Model file for the job. Use its own axes, mm. Coordinates: 2 decimals unless noted, no trailing zeros. Write each loop counter-clockwise with the first axis right and the second up, starting at its lowest first coordinate (ties: lowest second). Pieces come first, ordered by that corner, then holes. Notation, with made-up numbers: M 20,24.25 L 62,24.25 A35 cw 62,60.25 Z; hole C -2.75,87.25 d1. An arc over 180 degrees is marked long. Use CSV: the item, a comma, the result in double quotes. Start each with the question number.
from build123d import *

# Parameters (mm, degrees)
BOSS_EXTRUDE1_DEPTH                       = 3.175
CSK_FOR_0_FLAT_HEAD_MACHINE_SCREW_2_COUNT = 2
CSK_FOR_0_FLAT_HEAD_MACHINE_SCREW_2_PITCH = 47.625
LPATTERN1_COUNT                           = 4
LPATTERN1_PITCH                           = 25.4
LPATTERN2_COUNT                           = 3
LPATTERN2_PITCH                           = 50.8


with BuildPart() as part:
    # Sketch1 → Boss-Extrude1 (new body)
    with BuildSketch(Plane.XY):
        with BuildLine():
            Line((0, 0), (0, 152.4))
            Line((0, 152.4), (-6.35, 152.4))
            ThreePointArc((-6.35, 152.4), (-10.840128061, 154.259871939), (-12.7, 158.75))
            Line((-12.7, 158.75), (-12.7, 215.9))
            Line((-12.7, 215.9), (-129.54, 215.9))
            Line((-129.54, 215.9), (-129.54, 158.75))
            Line((-129.54, 158.75), (-44.45, 0))
            Line((-44.45, 0), (0, 0))
        make_face()
    extrude(amount=-BOSS_EXTRUDE1_DEPTH)

    # Sketch3 → CSK for _0 Flat Head Machine Screw _100 (revolve, cut)
    with BuildSketch(Plane(origin=(-114.3, 209.55, 0), x_dir=(0, -1, 0), z_dir=(1, 0, 0))):
        Polygon((0, 0), (0, 3.175), (2.7559, 3.175), (2.7559, 2.4384), (5.1943, 0), align=None)
    csk_for_0_flat_head_machine_screw_100 = revolve(axis=Axis((-114.3, 209.55, 6.35), (0, 0, -1)), mode=Mode.SUBTRACT)

    # CSK for _0 Flat Head Machine Screw _ 2: CSK for _0 Flat Head Machine Screw _100 ×2
    with Locations(*[(0, -i * CSK_FOR_0_FLAT_HEAD_MACHINE_SCREW_2_PITCH, 0) for i in range(1, CSK_FOR_0_FLAT_HEAD_MACHINE_SCREW_2_COUNT)]):
        add(csk_for_0_flat_head_machine_screw_100, mode=Mode.SUBTRACT)

    # LPattern1: CSK for _0 Flat Head Machine Screw _100 ×4
    with Locations(*[(i * LPATTERN1_PITCH, 0, 0) for i in range(1, LPATTERN1_COUNT)]):
        add(csk_for_0_flat_head_machine_screw_100, mode=Mode.SUBTRACT)

    # LPattern1 copy 1 sketch → LPattern1 copy 1 (revolve, cut)
    with BuildSketch(Plane(origin=(-88.9, 161.925, 0), x_dir=(0, -1, 0), z_dir=(1, 0, 0))):
        Polygon((0, 0), (0, 3.175), (2.7559, 3.175), (2.7559, 2.4384), (5.1943, 0), align=None)
    revolve(axis=Axis((-88.9, 161.925, 6.35), (0, 0, -1)), mode=Mode.SUBTRACT)

    # LPattern1 copy 2 sketch → LPattern1 copy 2 (revolve, cut)
    with BuildSketch(Plane(origin=(-63.5, 161.925, 0), x_dir=(0, -1, 0), z_dir=(1, 0, 0))):
        Polygon((0, 0), (0, 3.175), (2.7559, 3.175), (2.7559, 2.4384), (5.1943, 0), align=None)
    revolve(axis=Axis((-63.5, 161.925, 6.35), (0, 0, -1)), mode=Mode.SUBTRACT)

    # LPattern1 copy 3 sketch → LPattern1 copy 3 (revolve, cut)
    with BuildSketch(Plane(origin=(-38.1, 161.925, 0), x_dir=(0, -1, 0), z_dir=(1, 0, 0))):
        Polygon((0, 0), (0, 3.175), (2.7559, 3.175), (2.7559, 2.4384), (5.1943, 0), align=None)
    revolve(axis=Axis((-38.1, 161.925, 6.35), (0, 0, -1)), mode=Mode.SUBTRACT)

    # Sketch4 → CSK for _0 Flat Head Machine Screw _ 3 (revolve, cut)
    with BuildSketch(Plane(origin=(-15.875, 107.95, 0), x_dir=(0, -1, 0), z_dir=(1, 0, 0))):
        Polygon((0, 0), (0, 3.175), (2.7559, 3.175), (2.7559, 2.4384), (5.1943, 0), align=None)
    csk_for_0_flat_head_machine_screw_3 = revolve(axis=Axis((-15.875, 107.95, 6.35), (0, 0, -1)), mode=Mode.SUBTRACT)

    # LPattern2: CSK for _0 Flat Head Machine Screw _ 3 ×3
    with Locations(*[(0, -i * LPATTERN2_PITCH, 0) for i in range(1, LPATTERN2_COUNT)]):
        add(csk_for_0_flat_head_machine_screw_3, mode=Mode.SUBTRACT)


solid = part.part
1) Wall check: L1, parallel to Y at x = -38.1, z = -2.75; L2, parallel to X at y = 209.55, z = -2.75; L3, parallel to X at y = 194, z = -2.05. Give the ranges that are in metal, low to high. Write a range as [from, to].
2) Band-saw the part on D-D on y = 107.95. List the corners of the cut face in (x, z) (3 decimals), then the cut area to 3 significant figures.
3) Drop flat-ended pins along their axis: P1, Ø7, axis at x = -38.1, y = 161.925, coming from the +Z side; P2, Ø1.6, axis at x = -3.5, z = -2.5, coming from the +Y side; P3, Ø6.5, axis at x = -63.5, y = 161.925, coming from the +Z side. Give the stop position or say it passes through.
4) Band-saw the part on A-A on x = -38.1. List the corners of the cut face in (y, z) (3 decimals), then the cut area to 3 significant figures.
5) Band-saw the part on B-B on y = 6.35. List the corners of the cut face in (x, z) (3 decimals), then the cut area to 3 significant figures.
6) Two-plate mould, pull along X, no slides. Class faces 1 (the face through (-51, 109, 0)), 2 (the face through (-87.6, 80.5, -1.6)), 3 (the face through (-14.11, 8.66, -2.29)), 4 (the face through (-10.79, 154.21, -1.57)): pulls with the +X half, pulls with the -X half, needs draft (parallel to the pull), parting line crosses it, or undercut.
7) Band-saw the part on C-C on z = -1.6. State how many separate pieces and enclosed holes the cut face has, then the cut area to 3 significant figures.
Findings below:
1,L1,"y = [0, 159.17], [164.68, 206.79], [212.31, 215.9]"
1,L2,"x = [-129.54, -117.06], [-111.54, -91.66], [-86.14, -66.26], [-60.74, -40.86], [-35.34, -12.7]"
1,L3,"x = [-129.54, -12.7]"
2,outline,"M -102.311,-3.175 L -18.631,-3.175 L -18.631,-2.438 L -21.069,0 L -102.311,0 Z; M -13.119,-3.175 L 0,-3.175 L 0,0 L -10.681,0 L -13.119,-2.438 Z"
2,area,"301 mm2"
3,P1,"stops at z = -1.69"
3,P2,"stops at y = 152.4"
3,P3,"stops at z = -1.94"
4,outline,"M 0,-3.175 L 159.169,-3.175 L 159.169,-2.438 L 156.731,0 L 0,0 Z; M 164.681,-3.175 L 206.794,-3.175 L 206.794,-2.438 L 204.356,0 L 167.119,0 L 164.681,-2.438 Z; M 212.306,-3.175 L 215.9,-3.175 L 215.9,0 L 214.744,0 L 212.306,-2.438 Z"
4,area,"639 mm2"
5,outline,"M -47.854,-3.175 L -18.631,-3.175 L -18.631,-2.438 L -21.069,0 L -47.854,0 Z; M -13.119,-3.175 L 0,-3.175 L 0,0 L -10.681,0 L -13.119,-2.438 Z"
5,area,"128 mm2"
6,face 1,"needs draft"
6,face 2,"pulls with the -X half"
6,face 3,"undercut"
6,face 4,"pulls with the +X half"
7,separate pieces,"1"
7,enclosed holes,"11"
7,area,"20,000 mm2"
